Part model, mm, in its own coordinate system. A direction names the side the tool comes from. Round coordinates to 2 decimals unless told otherwise and drop trailing zeros. Loops run counter-clockwise (first coordinate to the right, second up) from the corner with the lowest first, then second, coordinate; pieces in that order, holes last. Notation, with made-up numbers: M 9,35.5 L 57,35.5 A23 ccw 57,50.5 Z; hole C 7.5,18.25 d6. An arc over 180 degrees is marked long. Put each result on its own line as item: value. Start each with the question number.
```python
from build123d import *

# Parameters (mm, degrees)
SKETCH_W     = 50
SKETCH_H     = 20
PAD_DEPTH    = 5
SKETCH001_R  = 2.5
PAD001_DEPTH = 3
SKETCH002_R  = 1
PAD002_DEPTH = 3


with BuildPart() as part:
    # Sketch → Pad (new body)
    with BuildSketch(Plane.XY):
        with Locations((25, 10)):
            Rectangle(SKETCH_W, SKETCH_H)
    extrude(amount=PAD_DEPTH)

    # Sketch001 (on Face6 of Pad) → Pad001 (join)
    with BuildSketch(Plane.XY.offset(5)):
        with Locations((5.5, 16.5)):
            Circle(SKETCH001_R)
        with Locations((36.916556, 3.5)):
            Circle(SKETCH001_R)
    extrude(amount=PAD001_DEPTH)

    # Sketch002 (on Face10 of Pad001) → Pad002 (join)
    with BuildSketch(Plane.XY.offset(8)):
        with Locations((5.5, 16.5)):
            Circle(SKETCH002_R)
        with Locations((36.916556, 3.5)):
            Circle(SKETCH002_R)
    extrude(amount=PAD002_DEPTH)


solid = part.part
```
1. Cut at A-A, the plane y = 18. Give the cut face in (x, z).
2. Cut at C-C, the plane x = 19.5. Give the cut face in (y, z).
3. Wall check: L1, parallel to Z at x = 24.5, y = 8.5; L2, parallel to X at y = 3.75, z = 8.25. Give the ranges that are in metal, low to high.
4. Cut at B-B, the plane x = 5.5. Give the cut face in (y, z).
5. Cut at D-D, the plane y = 12.25. Give the cut face in (x, z).
6. Which spindle directions (+Z, -Z, +X, -X, +Y, -Y) get a long thin tool onto all of the face, cutting with end or side? Do faces 1 (the flat face through (25, 0, 2)), 2 (the cylindrical face through (7.885, 17.251, 6.479)). Say none if no direction does.
7. Drop a flat-ended pin along its axis: pin 1 (8 mm diameter, centred on x = 13.5, y = 7, fed in from +Z). Give the stop position or say it passes through.
Results list:
1. outline: M 0,0 L 50,0 L 50,5 L 7.5,5 L 7.5,8 L 3.5,8 L 3.5,5 L 0,5 Z
2. outline: M 0,0 L 20,0 L 20,5 L 0,5 Z
3. L1: z = 0 to 5
3. L2: x = 35.95 to 37.88
4. outline: M 0,0 L 20,0 L 20,5 L 19,5 L 19,8 L 17.5,8 L 17.5,11 L 15.5,11 L 15.5,8 L 14,8 L 14,5 L 0,5 Z
5. outline: M 0,0 L 50,0 L 50,5 L 0,5 Z
6. face 1: +Z, -Z, +X, -X, -Y
6. face 2: +Z
7. pin 1: stops at z = 5
